Geometry check sheet. Reference: the model listing, model coordinates, mm. A direction names the side the tool comes from. Coordinates: 2 decimals unless noted, no trailing zeros. Write each loop counter-clockwise with the first axis right and the second up, starting at its lowest first coordinate (ties: lowest second). Pieces come first, ordered by that corner, then holes. Notation, with made-up numbers: (74.25, -32.5) -> (97.25, -32.5) arc R20 ccw to (97.25, -21.5) -> close; hole circle Ø7 at (-34, 88). An arc over 180 degrees is marked (long way). Answer in a Markdown table with one row per item. Add a question column.
Q1. Section check B-B, the plane x = 0. Count the separate pieces of the cut face and the enclosed holes in it, and give its area (3 significant figures).
Q2. Section check A-A, the plane z = 5.5. Record the boundary of the cut face in (x, y).
Q3. Release check for a two-part mould opening along Y. For faces 5 (the face through (-1.685, 5.38, 29.537)), 6 (the face through (3, 4, 33)) record: pulls with the +Y half, pulls with the -Y half, needs draft (parallel to the pull), parting line crosses it, or undercut.
Q4. Tool access check on faces 1 (the face through (-5.4, 1.67, 29.49)), 2 (the face through (0, 0, 10)), 3 (the face through (0, 15, 10)), 4 (the face through (-15, 0, 10)). Record the directions out of +Z, -Z, +X, -X, +Y, -Y that give a thin tool (end or side, any length) a straight path to the whole face; none if there is none.
Q5. Thickness scan on line 1 (Y direction, x = 0, z = 3.25); line 2 (X direction, y = -12, z = 28.5); line 3 (X direction, y = -2.5, z = 29.5). Record the ranges inside material, lowest first.
Q6. Gauge pin test, flat ends, axial feed: P1, Ø7.5, axis at x = 1.5, y = 14.5, coming from the +Z side; P2, Ø4, axis at y = 4, z = 28, coming from the -X side; P3, Ø10, axis at x = -12.5, z = 4, coming from the +Y side; P4, Ø1.9, axis at x = 13, y = 0, coming from the -Z side. Record the tip position at first contact, or that the pin passes through.
```python
from build123d import *

# Parameters (mm, degrees)
SKETCH1_R           = 17
BOSS_EXTRUDE1_DEPTH = 10
SKETCH2_R           = 1.55
CUT_EXTRUDE1_DEPTH  = 27.038433133
BOSS_EXTRUDE3_DEPTH = 23
SKETCH4_R           = 4
CUT_EXTRUDE2_DEPTH  = 23
SKETCH7_R           = 1.55
CUT_EXTRUDE3_DEPTH  = 15
CUT_EXTRUDE6_DEPTH  = 7


with BuildPart() as part:
    # Sketch1 → Boss-Extrude1 (new body)
    with BuildSketch(Plane.XY):
        Circle(SKETCH1_R)
    extrude(amount=BOSS_EXTRUDE1_DEPTH)

    # Sketch2 → Cut-Extrude1 (cut, through all)
    with BuildSketch(Plane.XY.offset(10)):
        with Locations((13, 0)):
            Circle(SKETCH2_R)
        with Locations((0, -13)):
            Circle(SKETCH2_R)
        with Locations((-13, 0)):
            Circle(SKETCH2_R)
        with Locations((0, 13)):
            Circle(SKETCH2_R)
    extrude(amount=-CUT_EXTRUDE1_DEPTH, mode=Mode.SUBTRACT)

    # Sketch3 → Boss-Extrude3 (add)
    with BuildSketch(Plane.XY.offset(10)):
        with BuildLine():
            ThreePointArc((16.522711642, 4), (12.02081528, 12.02081528), (4, 16.522711642))
            add(Edge.make_bspline(
                [(4, 16.522711642), (2.816233041, 15.179097537), (3.696027617, 11.190043266), (0, 9.66895733), (-3.696027617, 11.190043266), (-2.816233041, 15.179097537), (-4, 16.522711642)],
                knots=[0, 0, 0, 0, 0.360911498, 0.5, 0.639088502, 1, 1, 1, 1], degree=3))
            ThreePointArc((-4, 16.522711642), (-12.02081528, 12.02081528), (-16.522711642, 4))
            add(Edge.make_bspline(
                [(-16.522711642, 4), (-15.179097537, 2.816233041), (-11.190043266, 3.696027617), (-9.66895733, 0), (-11.190043266, -3.696027617), (-15.179097537, -2.816233041), (-16.522711642, -4)],
                knots=[0, 0, 0, 0, 0.360911498, 0.5, 0.639088502, 1, 1, 1, 1], degree=3))
            ThreePointArc((-16.522711642, -4), (-12.02081528, -12.02081528), (-4, -16.522711642))
            add(Edge.make_bspline(
                [(-4, -16.522711642), (-2.816233041, -15.179097537), (-3.696027617, -11.190043266), (0, -9.66895733), (3.696027617, -11.190043266), (2.816233041, -15.179097537), (4, -16.522711642)],
                knots=[0, 0, 0, 0, 0.360911498, 0.5, 0.639088502, 1, 1, 1, 1], degree=3))
            ThreePointArc((4, -16.522711642), (12.02081528, -12.02081528), (16.522711642, -4))
            add(Edge.make_bspline(
                [(16.522711642, -4), (15.179097537, -2.816233041), (11.190043266, -3.696027617), (9.66895733, 0), (11.190043266, 3.696027617), (15.179097537, 2.816233041), (16.522711642, 4)],
                knots=[0, 0, 0, 0, 0.360911498, 0.5, 0.639088502, 1, 1, 1, 1], degree=3))
        make_face()
    extrude(amount=BOSS_EXTRUDE3_DEPTH)

    # Sketch4 → Cut-Extrude2 (cut)
    with BuildSketch(Plane.XY.offset(33)):
        Circle(SKETCH4_R)
    extrude(amount=-CUT_EXTRUDE2_DEPTH, mode=Mode.SUBTRACT)

    # Sketch7 → Cut-Extrude3 (cut)
    with BuildSketch(Plane(origin=(-12.02081528, 12.02081528, 0), x_dir=(0, 0, -1), z_dir=(-0.7071067811865464, 0.7071067811865488, 0))):
        with Locations(Location((-28, 0, 0), (0, 0, 90))):
            Circle(SKETCH7_R)
    extrude(amount=-CUT_EXTRUDE3_DEPTH, mode=Mode.SUBTRACT)

    # Sketch11 → Cut-Extrude6 (cut)
    with BuildSketch(Plane(origin=(0, 0, 0), x_dir=(0, 0, -1), z_dir=(-0.7071067811865464, 0.7071067811865488, 0))):
        Polygon((-28, 3.5), (-31.031088913, 1.75), (-31.031088913, -1.75), (-28, -3.5), (-24.968911087, -1.75), (-24.968911087, 1.75), align=None)
    extrude(amount=CUT_EXTRUDE6_DEPTH, mode=Mode.SUBTRACT)


solid = part.part
```
Calculated:
| question | item | result |
|---|---|---|
| 1 | separate pieces | 3 |
| 1 | enclosed holes | 0 |
| 1 | area | 553 mm² |
| 2 | outline | circle Ø34 at (0, 0); hole circle Ø3.1 at (-13, 0); hole circle Ø3.1 at (0, -13); hole circle Ø3.1 at (0, 13); hole circle Ø3.1 at (13, 0) |
| 3 | face 5 | undercut |
| 3 | face 6 | needs draft |
| 4 | face 1 | none |
| 4 | face 2 | +Z |
| 4 | face 3 | +Z, +Y |
| 4 | face 4 | +Z, -X |
| 5 | line 1 | y = -17 to -14.55, -11.45 to 11.45, 14.55 to 17 |
| 5 | line 2 | x = -12.04 to -2.76, 2.76 to 12.04 |
| 5 | line 3 | x = -11.41 to -3.12, 3.12 to 11.41 |
| 6 | P1 | stops at z = 33 |
| 6 | P2 | stops at x = -16.52 |
| 6 | P3 | stops at y = 15.26 |
| 6 | P4 | passes through |
